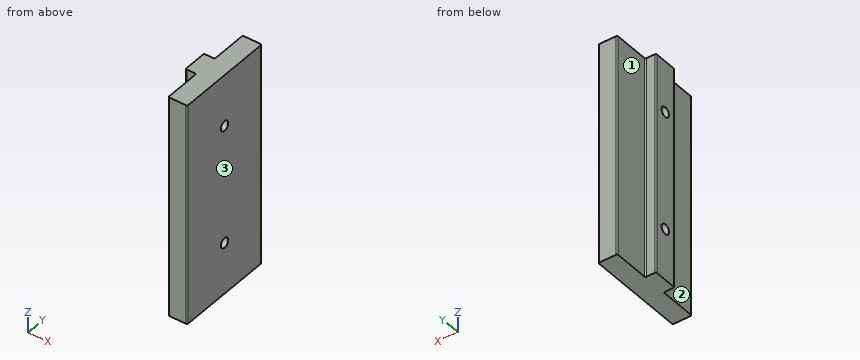
Autodesk Inventor part; units mm, degrees
ref_plane "p1_XY" through (6.096, 0, 19.05) normal (1, 0, 0) x (0, 0, -1)
ref_plane "p1_YZ" through (6.096, 0, 19.05) normal (0, 0, -1) x (0, 1, 0)
ref_plane "p1_ZX" through (6.096, 0, 19.05) normal (0, 1, 0) x (1, 0, 0)
sketch "Sketch_5" plane through (0, 0, 0) normal (0, 0, 1) x (1, 0, 0)
  line L0 (-3.429, 3.556) -> (-3.429, -3.556)
  arc A0 (-3.429, -3.556) -> (-3.048, -3.937) centre (-3.048, -3.556) ccw
  line L1 (-3.048, -3.937) -> (-0.381, -3.937)
  arc A1 (0, -4.318) -> (-0.381, -3.937) centre (-0.381, -4.318) ccw
  line L2 (0, -4.318) -> (0, -15.494)
  arc A2 (0, -15.494) -> (0.381, -15.875) centre (0.381, -15.494) ccw
  line L3 (0.381, -15.875) -> (5.715, -15.875)
  arc A3 (5.715, -15.875) -> (6.096, -15.494) centre (5.715, -15.494) ccw
  line L4 (6.096, -15.494) -> (6.096, 15.494)
  arc A4 (6.096, 15.494) -> (5.715, 15.875) centre (5.715, 15.494) ccw
  line L5 (5.715, 15.875) -> (0.381, 15.875)
  arc A5 (0.381, 15.875) -> (0, 15.494) centre (0.381, 15.494) ccw
  line L6 (0, 15.494) -> (0, 4.318)
  arc A6 (-0.381, 3.937) -> (0, 4.318) centre (-0.381, 4.318) ccw
  line L7 (-0.381, 3.937) -> (-3.048, 3.937)
  arc A7 (-3.048, 3.937) -> (-3.429, 3.556) centre (-3.048, 3.556) ccw
extrude "Extrusion1" add sketch "Sketch_5" along normal mid plane 71.12
sketch "Sketch2" plane through (6.096, -15.494, 35.56) normal (1, 0, 0) x (0, 0, -1)
  point P0 (16.51, 15.494)
hole "Hole1" at (6.096, 0, 19.05) direction (-1, 0, 0) diameter 3.175 depth 9.525
sketch "Sketch3" plane through (6.096, -15.494, 35.56) normal (1, 0, 0) x (0, 0, -1)
  point P0 (54.61, 15.494)
hole "Hole2" at (6.096, 0, -19.05) direction (-1, 0, 0) diameter 3.175 depth 9.525
ref_plane "p1_XY" through (6.096, 0, 19.05) normal (1, 0, 0) x (0, 0, -1)
ref_plane "p1_YZ" through (6.096, 0, 19.05) normal (0, 0, -1) x (0, 1, 0)
ref_plane "p1_ZX" through (6.096, 0, 19.05) normal (0, 1, 0) x (1, 0, 0)
properties part number "6825_p2"
Input: part model. Units: mm. Frame: model coordinates. Face numbers are marked on the shaded views. A direction names the side the tool comes from. Give positions to 0.01 mm unless a question says otherwise; leave off trailing zeros. Order: outer loops, then holes, each group sorted by start corner. A loop starts at its lowest first (then second) coordinate and runs counter-clockwise, first axis right, second up. Notation, with made-up numbers: M -37.75,11 L -27.75,11 A20 cw -27.75,42 Z; hole C -34,-14.75 d5. An arc over 180 degrees is marked long. Return JSON: item names as keys, results as strings.
1) Access query for the marked faces 1, 2 and 3. Directions: +Z, -Z, +X, -X, +Y, -Y. A direction counts if a zero-diameter tool reaches every point of the face in a straight line with its end or side. Return the directions, or none.
Taken from the geometry:
{"face 1": "+Z, -Z, -X, +Y", "face 2": "+Z, -Z, -X, -Y", "face 3": "+Z, -Z, +X, +Y, -Y"}
2) Section query B-B on y = 0. Output: boundary loops of the cut face in (x, z).
Taken from the geometry:
{"outline": "M -3.43,-35.56 L 6.1,-35.56 L 6.1,-20.64 L -3.43,-20.64 Z; M -3.43,-17.46 L 6.1,-17.46 L 6.1,17.46 L -3.43,17.46 Z; M -3.43,20.64 L 6.1,20.64 L 6.1,35.56 L -3.43,35.56 Z"}
3) Section query D-D on y = 11. Output: boundary loops of the cut face in (x, z).
Taken from the geometry:
{"outline": "M 0,-35.56 L 6.1,-35.56 L 6.1,35.56 L 0,35.56 Z"}
4) Section query A-A on z = -19.05. Output: boundary loops of the cut face in (x, y) (1 decimal).
Taken from the geometry:
{"outline": "M -3.4,-3.6 A0.4 ccw -3,-3.9 L -0.4,-3.9 A0.4 cw 0,-4.3 L 0,-15.5 A0.4 ccw 0.4,-15.9 L 5.7,-15.9 A0.4 ccw 6.1,-15.5 L 6.1,-1.6 L -3.4,-1.6 Z; M -3.4,1.6 L 6.1,1.6 L 6.1,15.5 A0.4 ccw 5.7,15.9 L 0.4,15.9 A0.4 ccw 0,15.5 L 0,4.3 A0.4 cw -0.4,3.9 L -3,3.9 A0.4 ccw -3.4,3.6 Z"}
5) Contact query for flat-ended pins moving along their axis: pin 1 (3 mm diameter, centred on y = 0, z = 19.05, fed in from -X); pin 2 (2 mm diameter, centred on x = -1.5, z = 12, fed in from +Y); pin 3 (5.5 mm diameter, centred on y = 11, z = -14, fed in from -X); pin 4 (3 mm diameter, centred on x = -2.5, z = -5.5, fed in from -Y). Output: stop coordinate, or through.
Taken from the geometry:
{"pin 1": "passes through", "pin 2": "stops at y = 3.94", "pin 3": "stops at x = 0", "pin 4": "stops at y = -3.94"}
6) Line query: L1, parallel to Z at x = 1.75, y = 0; L2, parallel to Y at x = 1.5, z = 19.05 (1 decimal); L3, parallel to Z at x = -1.75, y = 1. Output: solid intervals per line, ascending. Write a range as [from, to].
Taken from the geometry:
{"L1": "z = [-35.56, -20.64], [-17.46, 17.46], [20.64, 35.56]", "L2": "y = [-15.9, -1.6], [1.6, 15.9]", "L3": "z = [-35.56, -20.28], [-17.82, 17.82], [20.28, 35.56]"}
7) Section query C-C on x = -1.25. Count the separate pieces of the cut face and the enclosed holes in it, and give its area (3 significant figures).
Taken from the geometry:
{"separate pieces": "1", "enclosed holes": "2", "area": "544 mm2"}
